Study the drawing (mm; zero at the part's minimum x, y, z) and answer. A direction names the side the tool comes from. Give positions to 0.01 mm unless a question says otherwise; leave off trailing zeros. Write each loop counter-clockwise with the first axis right and the second up, starting at its lowest first coordinate (ties: lowest second). Pieces come first, ordered by that corner, then holes.
1) Straight lines are drawn through the part: probe 1 along Z at (x, y) = (28, 13.5); probe 2 along Z at (x, y) = (36.5, 49); probe 3 along X at (y, z) = (33, 29). For each, find the intervals that lie inside material, in ascending order.
2) Find section B-B (y = 40.5). Determine the outline of the cut face in (x, z) (1 decimal).
3) Find section D-D (y = 19.5). Determine the outline of the cut face in (x, z) (1 decimal), plus the area to 3 significant figures.
4) A tool of negligible diameter and unlimited length cuts with its end or side. For the marked faces 1, 2 and 3, from which of +Z, -Z, +X, -X, +Y, -Y can it reach the whole face along a straight path? Write none if from no direction.
5) Given pin 1 Ø4 at (x, z) = (19, 39) entering from +Y; pin 2 Ø0.9 at (x, y) = (21, 41) entering from -Z; pin 3 Ø5 at (x, y) = (21.38, 40.5) entering from +Z; pin 4 Ø8 at (y, z) = (55.5, 24) entering from +X, each flat-ended and moving along its own axis, determine where each tip first touches the part or whether it passes through.
6) Find section C-C (z = 35.5). Determine the outline of the cut face in (x, y), plus the area to 3 significant figures.
7) Find section A-A (z = 4). Determine the outline of the cut face in (x, y) (1 decimal).
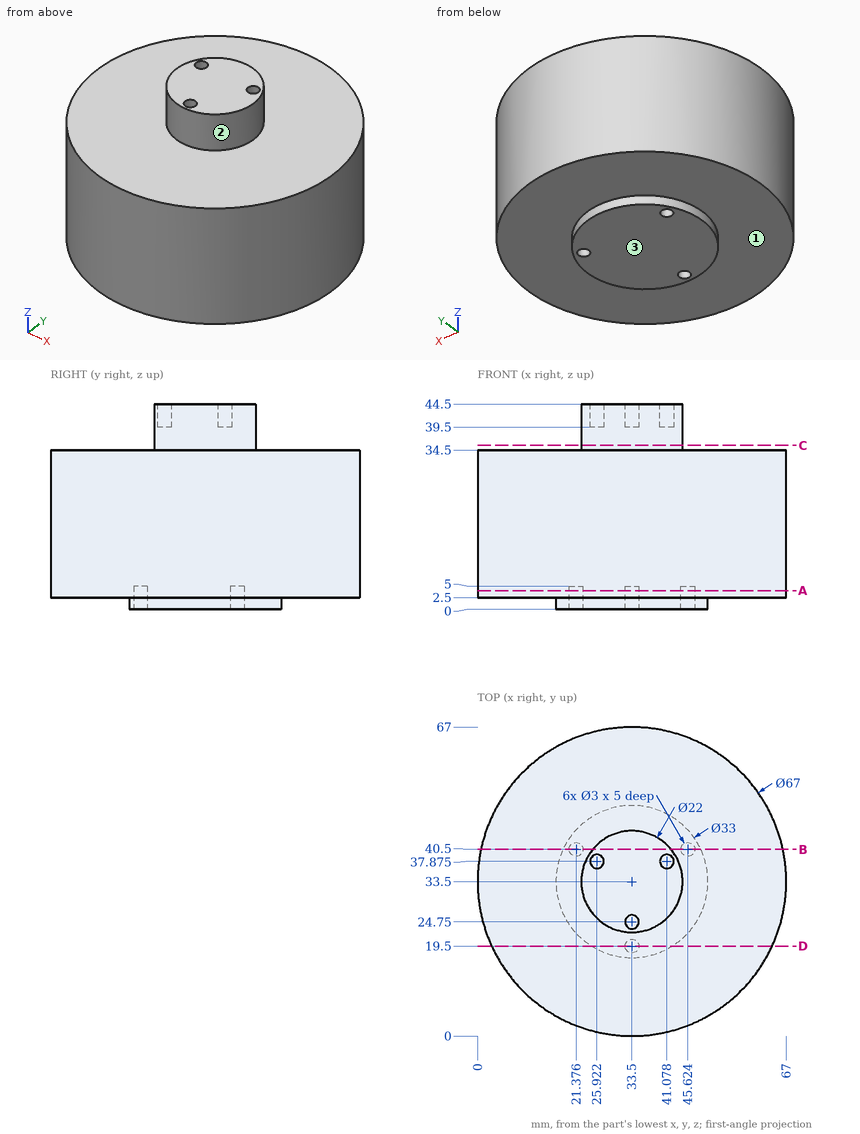
Results:
1. probe 1: z = 2.5 to 34.5
1. probe 2: z = 0 to 34.5
1. probe 3: x = 0 to 67
2. outline: (0.7, 2.5) - (18.6, 2.5) - (18.6, 0) - (19.9, 0) - (19.9, 5) - (22.9, 5) - (22.9, 0) - (44.1, 0) - (44.1, 5) - (47.1, 5) - (47.1, 0) - (48.4, 0) - (48.4, 2.5) - (66.3, 2.5) - (66.3, 34.5) - (42, 34.5) - (42, 44.5) - (25, 44.5) - (25, 34.5) - (0.7, 34.5) - close
3. outline: (3.1, 2.5) - (24.8, 2.5) - (24.8, 0) - (32, 0) - (32, 5) - (35, 5) - (35, 0) - (42.2, 0) - (42.2, 2.5) - (63.9, 2.5) - (63.9, 34.5) - (3.1, 34.5) - close
3. area: 1,980 mm2
4. face 1: -Z
4. face 2: +Z
4. face 3: -Z, +X, -X, +Y, -Y
5. pin 1: passes through
5. pin 2: stops at z = 5
5. pin 3: stops at z = 34.5
5. pin 4: stops at x = 61.75
6. outline: circle Ø22 at (33.5, 33.5)
6. area: 380 mm2
7. outline: circle Ø67 at (33.5, 33.5); hole circle Ø3 at (21.4, 40.5); hole circle Ø3 at (33.5, 19.5); hole circle Ø3 at (45.6, 40.5)
